from build123d import *

# Parameters (mm, degrees)
F1_DEPTH = 5
F2_W     = 19
F2_H     = 2.25
F3_DEPTH = 19
F4_W     = 19
F4_H     = 2.25
F5_DEPTH = 19


with BuildPart() as f1:
    # F0 (on Top) → F1 (new body)
    with BuildSketch(Plane.XY):
        with BuildLine():
            Line((-53.5, -83.5), (53.5, -83.5))
            ThreePointArc((53.5, -83.5), (74.713203, -74.713203), (83.5, -53.5))
            Line((83.5, -53.5), (83.5, 73.5))
            ThreePointArc((83.5, 73.5), (80.571068, 80.571068), (73.5, 83.5))
            Line((73.5, 83.5), (-73.5, 83.5))
            ThreePointArc((-73.5, 83.5), (-80.571068, 80.571068), (-83.5, 73.5))
            Line((-83.5, 73.5), (-83.5, -53.5))
            ThreePointArc((-83.5, -53.5), (-74.713203, -74.713203), (-53.5, -83.5))
        make_face()
    extrude(amount=F1_DEPTH)

    # F2 (on face) → F3 (join)
    with BuildSketch(Plane.XY.offset(5)):
        with Locations((0, -81)):
            Rectangle(F2_W, F2_H)
    extrude(amount=F3_DEPTH)

    # F4 (on face) → F5 (join)
    with BuildSketch(Plane.XY.offset(5)):
        with Locations((0, 81)):
            Rectangle(F4_W, F4_H)
    extrude(amount=F5_DEPTH)


solid = f1.part
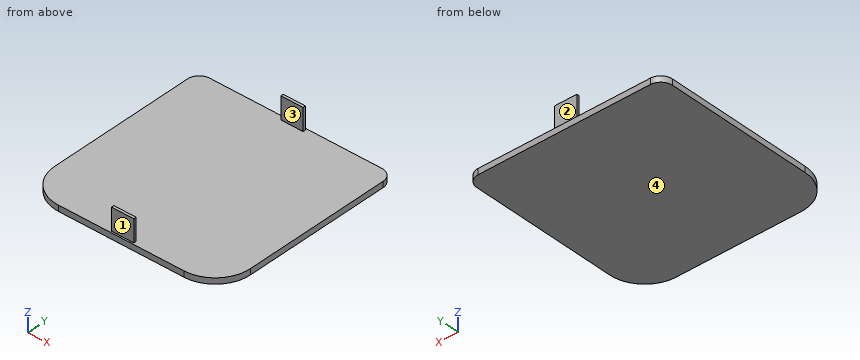
Work out the finished part from the listing and answer in its coordinate system (mm). Face numbers are marked on the shaded views. Coordinates: 2 decimals unless noted, no trailing zeros. Order: outer loops, then holes, each group sorted by start corner. A loop starts at its lowest first (then second) coordinate and runs counter-clockwise, first axis right, second up. Notation, with made-up numbers: (3.5, 32) - (54.5, 32) arc R6 ccw to (54.5, 43) - close; hole circle Ø11 at (32, -39). An arc over 180 degrees is marked (long way). Put each result on its own line as item: value. Start each with the question number.
1) Find section A-A (z = 9.25). Give the vertices of the cut face in (x, y) (3 decimals), plus the area to 3 significant figures.
2) Flat-ended cylindrical pins translate along their axes: pin 1 (0.7 mm diameter, centred on y = -81.5, z = 17, fed in from +X); pin 2 (8 mm diameter, centred on x = -36, y = 43, fed in from +Z); pin 3 (2.5 mm diameter, centred on y = 80.5, z = 16, fed in from -X). Find the tip coordinate at first contact, or state that the pin passes through.
3) For a pull along Y with two mould halves and no side action, classify the marked faces 1, 2, 3 and 4 as released by +Y, released by -Y, zero draft, split by the parting line, or undercut.
4) Find section B-B (x = -5). Give the vertices of the cut face in (y, z) (3 decimals), plus the area to 4 significant figures.
5) Find section C-C (y = -10). Give the vertices of the cut face in (x, z).
6) Find the intervals of material crossed by line 1 (Z direction, x = -5, y = 1); line 2 (Y direction, x = -59, z = 2), in increasing order. Write a range as from..to.
Results list:
1. outline: (-9.5, -82.125) - (9.5, -82.125) - (9.5, -79.875) - (-9.5, -79.875) - close; (-9.5, 79.875) - (9.5, 79.875) - (9.5, 82.125) - (-9.5, 82.125) - close
1. area: 85.5 mm^2
2. pin 1: stops at x = 9.5
2. pin 2: stops at z = 5
2. pin 3: stops at x = -9.5
3. face 1: released by -Y
3. face 2: released by +Y
3. face 3: undercut
3. face 4: zero draft
4. outline: (-83.5, 0) - (83.5, 0) - (83.5, 5) - (82.125, 5) - (82.125, 24) - (79.875, 24) - (79.875, 5) - (-79.875, 5) - (-79.875, 24) - (-82.125, 24) - (-82.125, 5) - (-83.5, 5) - close
4. area: 920.5 mm^2
5. outline: (-83.5, 0) - (83.5, 0) - (83.5, 5) - (-83.5, 5) - close
6. line 1: z = 0..5
6. line 2: y = -82.99..83.5
